Autodesk Fusion 360 part; units mm, degrees
sketch "Z main board" plane through (0, 0, 0) normal (0, 1, 0) x (1, 0, 0)
  circle A0 centre (89, -64) radius 3
  circle A1 centre (33, -7.5) radius 3.25
  circle A2 centre (-10, -109.5) radius 2.5
  line L0 (-71, -60) -> (-71, 150) construction
  line L1 (-80, -64) -> (100, -64) construction
  circle A3 centre (-71, -40.5) radius 3.25
  circle A4 centre (30, -133.4799) radius 2.5
  line L2 (45, -74.5) -> (-25, -74.5)
  line L3 (-70, -109.5) -> (80, -109.5) construction
  line L4 (45, -149.5) -> (45, -74.5)
  line L5 (-70, -133.5) -> (80, -133.5) construction
  line L6 (30, -133.4799) -> (30, -109.5) construction
  circle A5 centre (-35, -133.4853) radius 3
  circle A6 centre (55, -133.5) radius 3
  circle A7 centre (-35, -109.5) radius 3
  line L7 (91, -60) -> (91, 150) construction
  line L8 (-105, -149.5) -> (105, -149.5)
  line L9 (-80, -40.5) -> (100, -40.5) construction
  circle A8 centre (-69, -64) radius 3
  circle A9 centre (-13, -20.5) radius 3.25
  circle A10 centre (91, -40.5) radius 3.25
  line L10 (-20, -20.5) -> (45, -20.5) construction
  circle A11 centre (89, -96) radius 3
  line L11 (-13, -80) -> (-13, 145.5) construction
  line L12 (-105, 159.5) -> (-105, -149.5)
  circle A12 centre (-13, -7.5) radius 3.25
  line L13 (-69, -140) -> (-69, 140) construction
  line L14 (-39, -130) -> (-39, 150) construction
  circle A13 centre (-39, -96) radius 3
  circle A14 centre (-39, -64) radius 3
  circle A15 centre (30, -109.5) radius 2.5
  line L15 (59, -130) -> (59, 150) construction
  circle A16 centre (89, 99) radius 3
  line L16 (30, 13) -> (65, 13) construction
  line L17 (33, -80) -> (33, 145.5) construction
  circle A17 centre (59, 131) radius 3
  line L18 (89, 140) -> (89, -140) construction
  line L19 (35, -5) -> (35, 60) construction
  circle A18 centre (59, 53) radius 3
  line L20 (-80, 131) -> (100, 131) construction
  circle A19 centre (-69, 99) radius 3
  circle A20 centre (89, 131) radius 3
  line L21 (105, -149.5) -> (105, 159.5)
  circle A21 centre (59, 13) radius 3
  circle A22 centre (59, 145.5) radius 3.25
  circle A23 centre (35, 13) radius 3
  line L22 (105, 159.5) -> (-105, 159.5)
  line L23 (-80, 99) -> (100, 99) construction
  circle A24 centre (91, 145.5) radius 3.25
  circle A25 centre (-39, 145.5) radius 3.25
  circle A26 centre (-39, 99) radius 3
  circle A27 centre (33, 141.5) radius 3.25
  line L24 (30, 53) -> (65, 53) construction
  line L25 (-80, 145.5) -> (100, 145.5) construction
  circle A28 centre (-71, 145.5) radius 3.25
  line L26 (-20, 141.5) -> (40, 141.5) construction
  circle A29 centre (-69, 131) radius 3
  circle A30 centre (-39, 131) radius 3
  circle A31 centre (59, 99) radius 3
  circle A32 centre (35, 53) radius 3
  circle A33 centre (-13, 141.5) radius 3.25
  circle A34 centre (59, -64) radius 3
  circle A35 centre (59, -96) radius 3
  circle A36 centre (-39, -40.5) radius 3.25
  line L27 (-20, -7.5) -> (45, -7.5) construction
  line L28 (-80, -96) -> (100, -96) construction
  circle A37 centre (33, -20.5) radius 3.25
  line L29 (-25, -74.5) -> (-25, -149.5)
  line L30 (-10, -133.485) -> (-10, -109.5) construction
  line L31 (55, -134.9971) -> (55, -109.5) construction
  circle A38 centre (-10, -133.485) radius 2.5
  circle A39 centre (-69, -96) radius 3
  line L32 (-35, -133.4853) -> (-35, -109.5) construction
  circle A40 centre (59, -40.5) radius 3.25
  circle A41 centre (55, -109.5) radius 3
  line L33 (74, -32.219) -> (74, -146.1103) construction
  circle A42 centre (74, -80) radius 1
  circle A43 centre (74, -112) radius 1
  circle A44 centre (74, -140) radius 1
  dimension "d1" = 75
  dimension "d2" = 70
  dimension "d3" = 60
  dimension "d4" = 16
  dimension "d5" = 24
  dimension "d6" = 40
  dimension "d7" = 25
  dimension "d8" = 50
  dimension "d9" = 16
  dimension "d10" = 30
  dimension "d11" = 30
  dimension "d12" = 36
  dimension "d13" = 210
  dimension "d14" = 309
  dimension "d15" = 32
  dimension "d16" = 53.5
  dimension "d17" = 32
  dimension "d18" = 163
  dimension "d19" = 2
  dimension "d20" = 2
  dimension "d21" = 14.5
  dimension "d22" = 46
  dimension "d23" = 3
  dimension "d24" = 3
  dimension "d25" = 24
  dimension "d26" = 40
  dimension "d27" = 13
  dimension "d28" = 149
  dimension "d29" = 25
  dimension "d30" = 6
  dimension "d31" = 5
  dimension "d32" = 5
  dimension "d33" = 6
  dimension "d34" = 6
  dimension "d35" = 5
  dimension "d36" = 5
  dimension "d37" = 6
  dimension "d38" = 6
  dimension "d39" = 6
  dimension "d40" = 6
  dimension "d41" = 6
  dimension "d42" = 6
  dimension "d43" = 6
  dimension "d44" = 6
  dimension "d45" = 6
  dimension "d46" = 6
  dimension "d47" = 6
  dimension "d48" = 6
  dimension "d49" = 6
  dimension "d50" = 6
  dimension "d51" = 6
  dimension "d52" = 6
  dimension "d53" = 6
  dimension "d54" = 6.5
  dimension "d55" = 6.5
  dimension "d56" = 6.5
  dimension "d57" = 6.5
  dimension "d58" = 23.5
  dimension "d59" = 6.5
  dimension "d60" = 6.5
  dimension "d61" = 6.5
  dimension "d62" = 6.5
  dimension "d63" = 6.5
  dimension "d64" = 6.5
  dimension "d65" = 6.5
  dimension "d66" = 6.5
  dimension "d67" = 20
  dimension "d68" = 6.5
  dimension "d69" = 6.5
  dimension "d70" = 6
  dimension "d71" = 6
  dimension "d72" = 6
  dimension "d73" = 6
  dimension "d82" = 77
  dimension "d83" = 149
  dimension "d84" = 46
  dimension "d85" = 118
  dimension "d86" = 30
  dimension "d87" = 15
  dimension "d88" = 2
  dimension "d89" = 2
  dimension "d90" = 2
  dimension "d91" = 28
  dimension "d92" = 32
  dimension "d93" = 16
extrude "Extrude2" add sketch "Z main board" against normal blind 10 contours L2 L4 L8 L12 L21 L22 L29
extrude "Extrude3" add sketch "Z main board" against normal blind 4 contours L2 L4 L8 L29
extrude "Extrude4" add 1 faces at (-52.0966, -10, -17.5607) along direction (0, -1, 0) blind 8
equation "d87 = 30.0 mm / 2"
equation "d89 = d88"
equation "d90 = d88"
equation "d93 = d15 / 2"
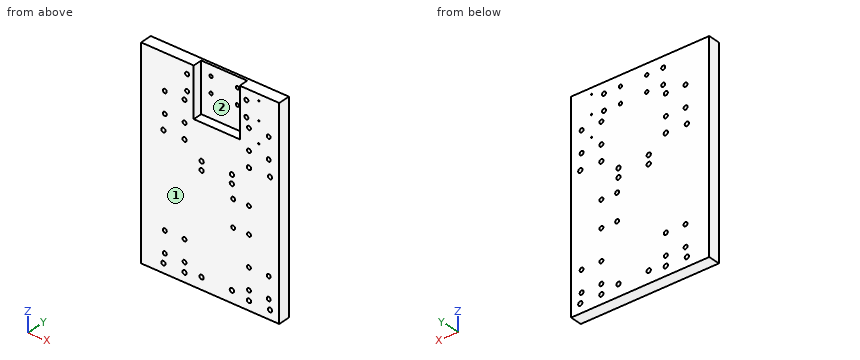
Input: part model. Units: mm. Frame: model coordinates. Face numbers are marked on the shaded views. Coordinates: 2 decimals unless noted, no trailing zeros. Order: outer loops, then holes, each group sorted by start corner. A loop starts at its lowest first (then second) coordinate and runs counter-clockwise, first axis right, second up. Notation, with made-up numbers: M 4,23.5 L 42,23.5 A4 cw 42,29.5 Z; hole C 47.5,-32.75 d5. An arc over 180 degrees is marked long. Write item = value, one per line. Start each with the question number.
(1) First-contact query: P1, Ø5, axis at x = 33, z = -141.5, coming from the +Y side; P2, Ø1.5, axis at x = 11.5, y = -5.5, coming from the +Z side. Flat tips, straight axial feed; report the tip coordinate or a pass-through.
(2) Pull-direction query (X, two-part tool) for the marked faces 1 and 2; classes: released by +X, released by -X, zero draft, split by the parting line, or undercut.
(3) Line query: line 1 along Z through (x, y) = (-13, -3.75); line 2 along Z through (x, y) = (74, -9.5); line 3 along X through (y, z) = (-14.5, 109.5). Output: solid intervals per line, ascending. Write a range as [from, to].
(4) Section B-B on x = 1.5. Output: boundary loops of the cut face in (y, z), and give its area (3 significant figures).
(5) Section C-C on y = -12.75. Give the number of separate pieces and of enclosed holes in the cut face, and give its area (3 significant figures).
(6) Section A-A on z = 88. Output: boundary loops of the cut face in (x, y), and give its area (3 significant figures).
Result set:
q1.P1 = through
q1.P2 = 74.5
q2.face_1 = zero draft
q2.face_2 = undercut
q3.line_1 = [-159.5, -144.75], [-138.25, 4.25], [10.75, 17.25], [23.75, 149.5]
q3.line_2 = [-159.5, 79], [81, 111], [113, 139], [141, 149.5]
q3.line_3 = [-105, -38], [-32, -25], [45, 52], [58, 105]
q4.outline = M -18,-159.5 L 0,-159.5 L 0,149.5 L -4,149.5 L -4,74.5 L -18,74.5 Z
q4.area = 4,510 mm²
q5.separate_pieces = 1
q5.enclosed_holes = 41
q5.area = 58,500 mm²
q6.outline = M -105,-18 L -25,-18 L -25,-4 L 45,-4 L 45,-18 L 105,-18 L 105,0 L -105,0 Z
q6.area = 2,800 mm²
